from build123d import *

# Parameters (mm, degrees)
BOSS_EXTRUDE1_DEPTH = 6.35


with BuildPart() as part:
    # Sketch1 → Boss-Extrude1 (new body, symmetric)
    with BuildSketch(Plane(origin=(0, 0, 0), x_dir=(0, 0, -1), z_dir=(1, 0, 0))):
        with BuildLine():
            Line((0, 19.05), (-3.175, 19.05))
            ThreePointArc((-3.175, 19.05), (-7.824679849, 7.824679849), (-19.05, 3.175))
            Line((-19.05, 3.175), (-19.05, 0))
            Line((-19.05, 0), (0, 0))
            Line((0, 0), (0, 19.05))
        make_face()
    extrude(amount=BOSS_EXTRUDE1_DEPTH, both=True)


solid = part.part
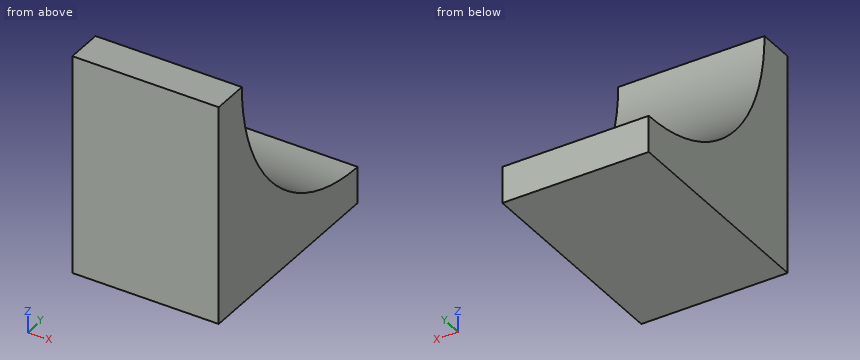
Here's how the part is built. I have some questions about the finished solid (model axes, mm). Coordinates: 2 decimals unless noted, no trailing zeros. Loops run counter-clockwise (first coordinate to the right, second up) from the corner with the lowest first, then second, coordinate; pieces in that order, holes last.
1. I need wall thicknesses on L1, parallel to Z at x = -4, y = 13.5; L2, parallel to Y at x = 4.25, z = 8.25; L3, parallel to Y at x = -5, z = 10.75. Which ranges of each line are inside material? Lowest first, please.
2. Imagine slicing it at A-A, the plane x = -4.5. Please give me the cut outline in (y, z) (3 decimals).
3. For P1, Ø5, axis at x = 4, y = 7.5, coming from the +Z side; P2, Ø3, axis at x = -4, y = 14.5, coming from the +Z side; P3, Ø8, axis at y = 6.5, z = 15, coming from the -X side; P4, Ø10, axis at y = 15, z = 10.5, coming from the +X side, each with a flat end and sliding along its axis, tell me the tip position at first contact or that it passes through.
4. Imagine slicing it at C-C, the plane z = 16.5. Please give me the cut outline in (x, y).
5. Imagine slicing it at B-B, the plane y = 14.5. Please give me the cut outline in (x, z).
Taken from the geometry:
1. L1: z = 0 to 4.18
1. L2: y = 0 to 7.41
1. L3: y = 0 to 5.52
2. outline: (0, 0) - (19.05, 0) - (19.05, 3.175) arc R15.875 cw to (3.175, 19.05) - (0, 19.05) - close
3. P1: stops at z = 11.66
3. P2: stops at z = 4.37
3. P3: stops at x = -6.35
3. P4: passes through
4. outline: (-6.35, 0) - (6.35, 0) - (6.35, 3.38) - (-6.35, 3.38) - close
5. outline: (-6.35, 0) - (6.35, 0) - (6.35, 3.84) - (-6.35, 3.84) - close
